```python
from build123d import *

# Parameters (mm, degrees)
ESBO_O1_W                = 60
ESBO_O1_H                = 110
ESBO_O1_R                = 1.75
RESSALTO_EXTRUS_O1_DEPTH = 6
ESBO_O2_R                = 1.75
CORTE_EXTRUS_O1_DEPTH    = 63.93647591
CORTE_EXTRUS_O3_DEPTH    = 63.93647591
FILETE1_R                = 5


with BuildPart() as part:
    # Esboço1 → Ressalto-extrusão1 (new body)
    with BuildSketch(Plane.XY):
        Rectangle(ESBO_O1_W, ESBO_O1_H)
        with Locations((23, -45)):
            Circle(ESBO_O1_R, mode=Mode.SUBTRACT)
        with Locations((23, -25)):
            Circle(ESBO_O1_R, mode=Mode.SUBTRACT)
        with Locations((3, -25)):
            Circle(ESBO_O1_R, mode=Mode.SUBTRACT)
    extrude(amount=RESSALTO_EXTRUS_O1_DEPTH)

    # Esboço2 → Corte-extrusão1 (cut, through all)
    with BuildSketch(Plane.XY.offset(6)):
        with Locations((-24, 49)):
            Circle(ESBO_O2_R)
        with Locations(Location((-3, 49, 0), (0, 0, 180))):
            Circle(ESBO_O2_R)
        with Locations((-13.5, 28)):
            Circle(ESBO_O2_R)
    extrude(amount=-CORTE_EXTRUS_O1_DEPTH, mode=Mode.SUBTRACT)

    # Esboço4 → Corte-extrusão3 (cut, through all)
    with BuildSketch(Plane(origin=(0, 0, 0), x_dir=(-1, 0, 0), z_dir=(0, 0, -1))):
        with BuildLine():
            Line((3, 54.75), (25.5, 54.75))
            ThreePointArc((25.5, 54.75), (28.681980515, 53.431980515), (30, 50.25))
            Line((30, 50.25), (30, 18.54785582))
            Line((30, 18.54785582), (51.213466558, 18.54785582))
            Line((51.213466558, 18.54785582), (51.213466558, 63.658711058))
            Line((51.213466558, 63.658711058), (-45.570141277, 63.658711058))
            Line((-45.570141277, 63.658711058), (-45.570141277, -25))
            Line((-45.570141277, -25), (-30, -25))
            Line((-30, -25), (-2.404439279, 50.963297246))
            ThreePointArc((-2.404439279, 50.963297246), (-0.299510633, 53.709111337), (3, 54.75))
        make_face()
    extrude(amount=-CORTE_EXTRUS_O3_DEPTH, mode=Mode.SUBTRACT)

    # Filete1
    filete1_edges = [part.edges().sort_by_distance(p)[0] for p in [
        (30, -25, 3),
        (30, -55, 3),
        (-30, -55, 3),
    ]]
    fillet(filete1_edges, radius=FILETE1_R)


solid = part.part
```
Here's how the part is built. I have some questions about the finished solid (model axes, mm). Give positions to 0.01 mm unless a question says otherwise; leave off trailing zeros. Order: outer loops, then holes, each group sorted by start corner. A loop starts at its lowest first (then second) coordinate and runs counter-clockwise, first axis right, second up. Notation, with made-up numbers: (-38, 66.25) - (-24, 66.25) arc R28 cw to (-24, 103.25) - close; hole circle Ø3 at (-6, 13). An arc over 180 degrees is marked (long way). Answer as a JSON object with one key per item and string values. Group by question number.
Item 1: For P1, Ø3, axis at x = -3, y = 49, coming from the +Z side, with a flat end and sliding along its axis, tell me the tip position at first contact or that it passes through.
Item 2: If we section it at B-B on y = -45: Please give me the cut outline in (x, z).
Item 3: Please list where these lines run through material, in increasing order: probe 1 along Y at (x, z) = (-24, 4.6); probe 2 along X at (y, z) = (41, 2.25); probe 3 along Y at (x, z) = (-23, 3.15).
Item 4: If we section it at A-A on x = -13.5: Please give me the cut outline in (y, z), and give its area (4 significant figures).
Item 5: If we mould it in two halves opening along Y, with no side actions, what happens to faces 1 (the cylindrical face through (21.71, -23.82, 2.96)), 2 (the flat face through (-14, 54.75, 3)), 3 (the flat face through (-7, 1, 6))? For each: pulls with the +Y half, pulls with the -Y half, needs draft (parallel to the pull), parting line crosses it, or undercut.
Item 6: If we section it at C-C on z = 2.6: Please give me the cut outline in (x, y), and give its area (3 significant figures).
Item 7: If we section it at D-D on y = 49: Please give me the cut outline in (x, z).
Result set:
{
 "1": {"P1": "through"},
 "2": {"outline": "(-30, 0) - (21.25, 0) - (21.25, 6) - (-30, 6) - close; (24.75, 0) - (30, 0) - (30, 6) - (24.75, 6) - close"},
 "3": {"probe 1": "-55 to 47.25, 50.75 to 54.75", "probe 2": "-30 to 6.02", "probe 3": "-55 to 47.56, 50.44 to 54.75"},
 "4": {"outline": "(-55, 0) - (26.25, 0) - (26.25, 6) - (-55, 6) - close; (29.75, 0) - (54.75, 0) - (54.75, 6) - (29.75, 6) - close", "area": "637.5 mm²"},
 "5": {"face 1": "undercut", "face 2": "pulls with the +Y half", "face 3": "needs draft"},
 "6": {"outline": "(-30, -50) arc R5 ccw to (-25, -55) - (25, -55) arc R5 ccw to (30, -50) - (30, -25.88) arc R5 ccw to (29.7, -24.17) - (2.4, 50.96) arc R5.75 ccw to (-3, 54.75) - (-25.5, 54.75) arc R4.5 ccw to (-30, 50.25) - close; hole circle Ø3.5 at (-24, 49); hole circle Ø3.5 at (-13.5, 28); hole circle Ø3.5 at (-3, 49); hole circle Ø3.5 at (3, -25); hole circle Ø3.5 at (23, -45); hole circle Ø3.5 at (23, -25)", "area": "5,350 mm²"},
 "7": {"outline": "(-30, 0) - (-25.75, 0) - (-25.75, 6) - (-30, 6) - close; (-22.25, 0) - (-4.75, 0) - (-4.75, 6) - (-22.25, 6) - close; (-1.25, 0) - (3.12, 0) - (3.12, 6) - (-1.25, 6) - close"}
}
